Part model, mm, in its own coordinate system. A direction names the side the tool comes from. Round coordinates to 2 decimals unless told otherwise and drop trailing zeros. Write each loop counter-clockwise with the first axis right and the second up, starting at its lowest first coordinate (ties: lowest second). Pieces come first, ordered by that corner, then holes. Notation, with made-up numbers: (-33, 85) -> (6, 85) arc R26 ccw to (6, 124) -> close; hole circle Ø7 at (58, -15). An arc over 180 degrees is marked (long way). Use CSV: the item, a comma, the result in double quotes. Start each with the question number.
(1) Saw through at A-A (x = 0). Give the cut face in (y, z), plus the area to 3 significant figures.
(2) Which spindle directions (+Z, -Z, +X, -X, +Y, -Y) get a long thin tool onto all of the face, cutting with end or side? Do faces 1 (the flat face through (36.805, 7.685, 2.06)), 2 (the flat face through (-2, 20, 14.986)), 3 (the cylindrical face through (17.74, 13.6, 9.45)). Say none if no direction does.
(3) Saw through at D-D (y = -43.5). Give the cut face in (x, z).
(4) Two-plate mould, pull along X, no slides. Class faces 4 (the flat face through (4.064, 37, 2)), 5 (the flat face through (-11, 11, 0)), 6 (the cylindrical face through (11.508, 51.824, 2.004)): released by +X, released by -X, zero draft, split by the parting line, or undercut.
(5) Saw through at B-B (y = 0). Give the cut face in (x, z), plus the area to 3 significant figures.
(6) Saw through at C-C (z = 5.75). Give the cut face in (x, y), plus the area to 3 significant figures.
(7) Drop flat-ended pins along their axis: pin 1 (8 mm diameter, centred on y = 16, z = 3, fed in from +X); pin 2 (3.5 mm diameter, centred on x = 0, y = 48.514, fed in from -Z); pin 3 (1.2 mm diameter, centred on y = 33.5, z = 2.5, fed in from -X); pin 4 (4 mm diameter, centred on y = -11, z = 9, fed in from +X). Give the stop position or say it passes through.
(8) Probe line 1 (Y direction, x = 0, z = 3.5); line 2 (X direction, y = -35.5, z = 2.25); line 3 (Y direction, x = 0, z = 4.5). List the from-to ranges inside material, lowest first. Write a range as [from, to].
```python
from build123d import *

# Parameters (mm, degrees)
SKETCH2_R          = 2.032
CUT_EXTRUDE1_DEPTH = 76.865254735
CIRPATTERN1_COUNT  = 5


with BuildPart() as part:
    # Sketch1 → Revolve1 (revolve)
    with BuildSketch(Plane(origin=(0, 0, 0), x_dir=(0, 0, -1), z_dir=(1, 0, 0)), mode=Mode.PRIVATE) as revolve1_sk:
        Polygon((0, 14.986), (-9.398, 14.986), (-9.398, 19.812), (-14.986, 19.812), (-14.986, 22.352), (-4.064, 22.352), (-4.064, 53.086), (0, 53.086), align=None)
    revolve(revolve1_sk.sketch.rotate(Axis((0, 0, 0), (0, 0, 1)), 90), axis=Axis((0, 0, 0), (0, 0, 1)))

    # Sketch2 → Cut-Extrude1 (cut, through all)
    with BuildSketch(Plane.XY.offset(4.064)):
        with Locations((0, 48.514)):
            Circle(SKETCH2_R)
        with BuildLine():
            Line((4.064, 48.343480429), (4.064, 26.1015126))
            ThreePointArc((4.064, 26.1015126), (15.526935225, 21.370992923), (23.568168578, 11.930904654))
            Line((23.568168578, 11.930904654), (44.721537017, 18.804050702))
            ThreePointArc((44.721537017, 18.804050702), (28.51581373, 39.248650465), (4.064, 48.343480429))
        make_face()
    cut_extrude1 = extrude(amount=-CUT_EXTRUDE1_DEPTH, mode=Mode.SUBTRACT)

    # CirPattern1: Cut-Extrude1 ×5 about axis
    cirpattern1_axis = Axis((0, 0, 0), (0, 0, 1))
    for i in range(1, CIRPATTERN1_COUNT):
        add(cut_extrude1.rotate(cirpattern1_axis, i * 360 / CIRPATTERN1_COUNT), mode=Mode.SUBTRACT)


solid = part.part
```
Answers:
1,outline,"(-53.09, 0) -> (-48.51, 0) -> (-48.51, 4.06) -> (-53.09, 4.06) -> close; (-26.42, 0) -> (-14.99, 0) -> (-14.99, 9.4) -> (-19.81, 9.4) -> (-19.81, 14.99) -> (-22.35, 14.99) -> (-22.35, 4.06) -> (-26.42, 4.06) -> close; (14.99, 0) -> (46.48, 0) -> (46.48, 4.06) -> (22.35, 4.06) -> (22.35, 14.99) -> (19.81, 14.99) -> (19.81, 9.4) -> (14.99, 9.4) -> close; (50.55, 0) -> (53.09, 0) -> (53.09, 4.06) -> (50.55, 4.06) -> close"
1,area,"310 mm²"
2,face 1,"+Z, -Z"
2,face 2,"+Z, +X, -X, +Y, -Y"
2,face 3,"+Z"
3,outline,"(-30.43, 0) -> (-21.48, 0) -> (-21.48, 4.06) -> (-30.43, 4.06) -> close; (21.48, 0) -> (30.43, 0) -> (30.43, 4.06) -> (21.48, 4.06) -> close"
4,face 4,"undercut"
4,face 5,"zero draft"
4,face 6,"split by the parting line"
5,outline,"(-53.09, 0) -> (-48.51, 0) -> (-48.51, 4.06) -> (-53.09, 4.06) -> close; (-26.42, 0) -> (-14.99, 0) -> (-14.99, 9.4) -> (-19.81, 9.4) -> (-19.81, 14.99) -> (-22.35, 14.99) -> (-22.35, 4.06) -> (-26.42, 4.06) -> close; (14.99, 0) -> (26.42, 0) -> (26.42, 4.06) -> (22.35, 4.06) -> (22.35, 14.99) -> (19.81, 14.99) -> (19.81, 9.4) -> (14.99, 9.4) -> close; (48.51, 0) -> (53.09, 0) -> (53.09, 4.06) -> (48.51, 4.06) -> close"
5,area,"237 mm²"
6,outline,"circle Ø44.7 at (0, 0); hole circle Ø29.97 at (0, 0)"
6,area,"864 mm²"
7,pin 1,"stops at x = 51.71"
7,pin 2,"passes through"
7,pin 3,"stops at x = -41.66"
7,pin 4,"stops at x = 20.46"
8,line 1,"y = [-53.09, -48.51], [-26.42, -14.99], [14.99, 46.48], [50.55, 53.09]"
8,line 2,"x = [-39.47, -33.07], [-30.82, -20.77], [20.77, 30.82], [33.07, 39.47]"
8,line 3,"y = [-22.35, -14.99], [14.99, 22.35]"
